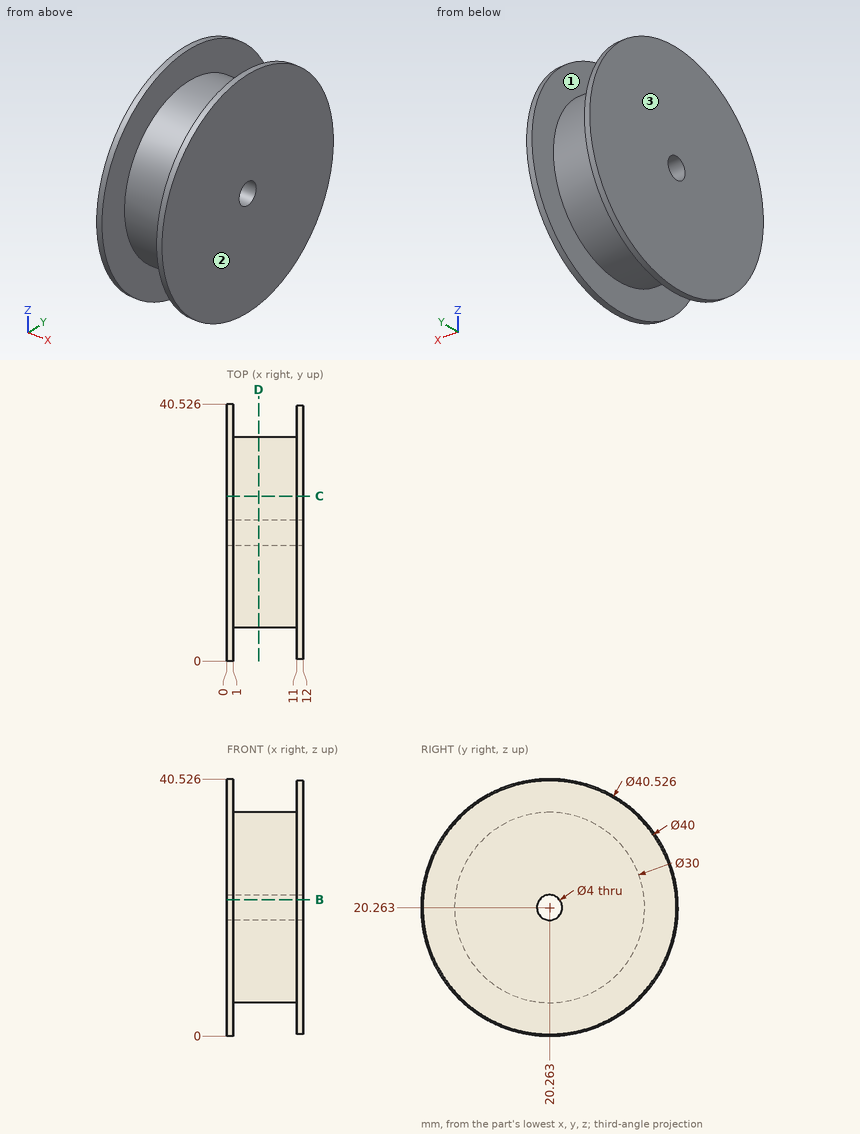
Geometry: see drawing. Coordinates: mm, zero at the bounding-box minimum. Give positions to 0.01 mm unless a question says otherwise; leave off trailing zeros. Order: outer loops, then holes, each group sorted by start corner. A loop starts at its lowest first (then second) coordinate and runs counter-clockwise, first axis right, second up. Notation, with made-up numbers: M 85,-9.75 L 106,-9.75 A25 ccw 106,13.25 Z; hole C 74.5,-11 d8. An arc over 180 degrees is marked long. Answer as CSV lines item,"result". Start each with the question number.
1) Line query: line 1 (X direction, y = 7.5, z = 6); line 2 (Y direction, x = 5.25, z = 29) (1 decimal); line 3 (Z direction, x = 7, y = 27) (1 decimal). Output: solid intervals per line, ascending. Write a range as from..to.
2) First-contact query: P1, Ø5, axis at x = 7, y = 6, coming from the -Z side (1 decimal); P2, Ø1, axis at x = 8, z = 13, coming from the -Y side (1 decimal); P3, Ø2, axis at x = 6, z = 29.5, coming from the +Y side. Flat tips, straight axial feed; report the tip coordinate or a pass-through.
3) Mould query, pull axis X, two halves, no side actions, for the marked faces 1, 2 and 3. Classes: +X half, -X half, draft (parallel to the pull), parting line (faces both ways), or undercut.
4) Cut plane C-C (y = 26). Output: boundary loops of the cut face in (x, z).
5) Cut plane B-B (z = 21.5). Output: boundary loops of the cut face in (x, y) (1 decimal).
6) Cut plane D-D (x = 5). Output: boundary loops of the cut face in (y, z).
Findings below:
1,line 1,"x = 0..1, 11..12"
1,line 2,"y = 8.1..32.5"
1,line 3,"z = 6.9..33.7"
2,P1,"stops at z = 11"
2,P2,"stops at y = 6.9"
2,P3,"stops at y = 32.8"
3,face 1,"undercut"
3,face 2,"+X half"
3,face 3,"-X half"
4,outline,"M 0,0.83 L 1,0.83 L 1,6.4 L 11,6.4 L 11,1.1 L 12,1.1 L 12,39.42 L 11,39.42 L 11,34.12 L 1,34.12 L 1,39.7 L 0,39.7 Z"
5,outline,"M 0,0 L 1,0 L 1,5.3 L 11,5.3 L 11,0.3 L 12,0.3 L 12,18.7 L 0,18.7 Z; M 0,21.8 L 12,21.8 L 12,40.2 L 11,40.2 L 11,35.2 L 1,35.2 L 1,40.5 L 0,40.5 Z"
6,outline,"C 20.26,20.26 d30; hole C 20.26,20.26 d4"
